Verification items for the finished model (mm, model axes). A direction names the side the tool comes from. Round coordinates to 2 decimals unless told otherwise and drop trailing zeros. Order: outer loops, then holes, each group sorted by start corner. A loop starts at its lowest first (then second) coordinate and runs counter-clockwise, first axis right, second up.
```python
from build123d import *

# Parameters (mm, degrees)
SKETCH_1_W          = 10
SKETCH_1_H          = 10
SKETCH_1_W_2        = 8
SKETCH_1_H_2        = 8
EXTRUDE_1_DEPTH     = 150
SKETCH_2_R          = 1.5
CUT_EXTRUDE_1_DEPTH = 11
SKETCH_3_R          = 1.5
CUT_EXTRUDE_2_DEPTH = 11


with BuildPart() as part:
    # 草图1 → 拉伸-薄壁1 (new body)
    with BuildSketch(Plane.XY):
        with Locations((4.161089293, -159.112745336)):
            Rectangle(SKETCH_1_W, SKETCH_1_H)
        with Locations((4.161089293, -159.112745336)):
            Rectangle(SKETCH_1_W_2, SKETCH_1_H_2, mode=Mode.SUBTRACT)
    extrude(amount=EXTRUDE_1_DEPTH)

    # 草图2 → 切除-拉伸1 (cut, through all)
    with BuildSketch(Plane.XZ.offset(164.112745336)):
        with Locations((4.161089293, 135)):
            Circle(SKETCH_2_R)
        with Locations((4.161089293, 66)):
            Circle(SKETCH_2_R)
        with Locations((4.161089293, 5)):
            Circle(SKETCH_2_R)
    extrude(amount=-CUT_EXTRUDE_1_DEPTH, mode=Mode.SUBTRACT)

    # 草图3 → 切除-拉伸2 (cut, through all)
    with BuildSketch(Plane(origin=(9.161089293, 0, 0), x_dir=(0, 0, -1), z_dir=(1, 0, 0))):
        with Locations((-25, -159.112745336)):
            Circle(SKETCH_3_R)
        with Locations((-10, -159.112745336)):
            Circle(SKETCH_3_R)
        with Locations((-120, -159.112745336)):
            Circle(SKETCH_3_R)
        with Locations((-145, -159.112745336)):
            Circle(SKETCH_3_R)
    extrude(amount=-CUT_EXTRUDE_2_DEPTH, mode=Mode.SUBTRACT)


solid = part.part
```
1) Sectioned sample at C-C on z = 128. Record the cut outline in (x, y), then the cut area to 3 significant figures.
2) Draft check along Y on faces 3 (the flat face through (4.1, -163.5, 150)), 4 (the flat face through (4, -154.113, 74)), 5 (the cylindrical face through (8.668, -160.577, 25.325)). Enter one of: released by +Y, released by -Y, zero draft, split by the parting line, or undercut.
3) Sectioned sample at B-B on x = 4.25. Count the separate pieces of the cut face and the enclosed holes in it, then the cut area to 3 significant figures.
4) Sectioned sample at A-A on z = 145. Record the cut outline in (x, y).
5) Scan lines: probe 1 along Y at (x, z) = (4.25, 122); probe 2 along X at (y, z) = (-162.5, 95.5); probe 3 along Y at (x, z) = (8.7, 120). Record each from-to range of solid material in increasing order.
6) Tool access check on faces 1 (the cylindrical face through (8.668, -160.577, 145.325)), 2 (the flat face through (0.161, -159, 74)). Record the directions out of +Z, -Z, +X, -X, +Y, -Y that give a thin tool (end or side, any length) a straight path to the whole face; none if there is none.
Returned:
1. outline: (-0.84, -164.11) - (9.16, -164.11) - (9.16, -154.11) - (-0.84, -154.11) - close; hole (0.16, -163.11) - (8.16, -163.11) - (8.16, -155.11) - (0.16, -155.11) - close
1. area: 36.0 mm2
2. face 3: zero draft
2. face 4: released by +Y
2. face 5: undercut
3. separate pieces: 8
3. enclosed holes: 0
3. area: 282 mm2
4. outline: (-0.84, -164.11) - (9.16, -164.11) - (9.16, -160.61) - (8.16, -160.61) - (8.16, -163.11) - (0.16, -163.11) - (0.16, -160.61) - (-0.84, -160.61) - close; (-0.84, -157.61) - (0.16, -157.61) - (0.16, -155.11) - (8.16, -155.11) - (8.16, -157.61) - (9.16, -157.61) - (9.16, -154.11) - (-0.84, -154.11) - close
5. probe 1: y = -164.11 to -163.11, -155.11 to -154.11
5. probe 2: x = -0.84 to 0.16, 8.16 to 9.16
5. probe 3: y = -164.11 to -160.61, -157.61 to -154.11
6. face 1: +X, -X
6. face 2: +Z, -Z
